```python
from build123d import *

# Parameters (mm, degrees)
SKETCH1_W           = 260
SKETCH1_H           = 170
BOSS_EXTRUDE1_DEPTH = 2
BOSS_EXTRUDE2_DEPTH = 3
CUT_EXTRUDE1_DEPTH  = 156.402702679
SKETCH4_R           = 2.5
CUT_EXTRUDE2_DEPTH  = 156.402702679
CUT_EXTRUDE3_REACH  = 157.403
SKETCH6_R           = 2.25


with BuildPart() as part:
    # Sketch1 → Boss-Extrude1 (new body)
    with BuildSketch(Plane.XY):
        Rectangle(SKETCH1_W, SKETCH1_H)
    extrude(amount=BOSS_EXTRUDE1_DEPTH)

    # Sketch2 → Boss-Extrude2 (add)
    with BuildSketch(Plane(origin=(0, 0, 0), x_dir=(-1, 0, 0), z_dir=(0, 0, -1))):
        with BuildLine():
            Line((-120.492, 81.492), (120.492, 81.492))
            Line((120.492, 81.492), (120.492, 79))
            ThreePointArc((120.492, 79), (121.519469412, 76.519469412), (124, 75.492))
            Line((124, 75.492), (126.492, 75.492))
            Line((126.492, 75.492), (126.492, -75.492))
            Line((126.492, -75.492), (124, -75.492))
            ThreePointArc((124, -75.492), (121.519469412, -76.519469412), (120.492, -79))
            Line((120.492, -79), (120.492, -81.492))
            Line((120.492, -81.492), (-120.492, -81.492))
            Line((-120.492, -81.492), (-120.492, -79))
            ThreePointArc((-120.492, -79), (-121.519469412, -76.519469412), (-124, -75.492))
            Line((-124, -75.492), (-126.492, -75.492))
            Line((-126.492, -75.492), (-126.492, 75.492))
            Line((-126.492, 75.492), (-124, 75.492))
            ThreePointArc((-124, 75.492), (-121.519469412, 76.519469412), (-120.492, 79))
            Line((-120.492, 79), (-120.492, 81.492))
        make_face()
    extrude(amount=BOSS_EXTRUDE2_DEPTH)

    # Sketch3 → Cut-Extrude1 (cut, through all)
    with BuildSketch(Plane.XY.offset(2)):
        with BuildLine():
            Line((-108.441183291, -1.769742849), (-108.441183291, -51.769742849))
            ThreePointArc((-108.441183291, -51.769742849), (-109.941183291, -53.269742849), (-111.441183291, -51.769742849))
            Line((-111.441183291, -51.769742849), (-111.441183291, -1.769742849))
            ThreePointArc((-111.441183291, -1.769742849), (-109.941183291, -0.269742849), (-108.441183291, -1.769742849))
        make_face()
        with BuildLine():
            Line((-103.441183291, -1.769742849), (-103.441183291, -51.769742849))
            ThreePointArc((-103.441183291, -51.769742849), (-104.941183291, -53.269742849), (-106.441183291, -51.769742849))
            Line((-106.441183291, -51.769742849), (-106.441183291, -1.769742849))
            ThreePointArc((-106.441183291, -1.769742849), (-104.941183291, -0.269742849), (-103.441183291, -1.769742849))
        make_face()
        with BuildLine():
            Line((-98.441183291, -1.769742849), (-98.441183291, -51.769742849))
            ThreePointArc((-98.441183291, -51.769742849), (-99.941183291, -53.269742849), (-101.441183291, -51.769742849))
            Line((-101.441183291, -51.769742849), (-101.441183291, -1.769742849))
            ThreePointArc((-101.441183291, -1.769742849), (-99.941183291, -0.269742849), (-98.441183291, -1.769742849))
        make_face()
        with BuildLine():
            Line((-93.441183291, -1.769742849), (-93.441183291, -51.769742849))
            ThreePointArc((-93.441183291, -51.769742849), (-94.941183291, -53.269742849), (-96.441183291, -51.769742849))
            Line((-96.441183291, -51.769742849), (-96.441183291, -1.769742849))
            ThreePointArc((-96.441183291, -1.769742849), (-94.941183291, -0.269742849), (-93.441183291, -1.769742849))
        make_face()
        with BuildLine():
            Line((-88.441183291, -1.769742849), (-88.441183291, -51.769742849))
            ThreePointArc((-88.441183291, -51.769742849), (-89.941183291, -53.269742849), (-91.441183291, -51.769742849))
            Line((-91.441183291, -51.769742849), (-91.441183291, -1.769742849))
            ThreePointArc((-91.441183291, -1.769742849), (-89.941183291, -0.269742849), (-88.441183291, -1.769742849))
        make_face()
        with BuildLine():
            Line((-83.441183291, -1.769742849), (-83.441183291, -51.769742849))
            ThreePointArc((-83.441183291, -51.769742849), (-84.941183291, -53.269742849), (-86.441183291, -51.769742849))
            Line((-86.441183291, -51.769742849), (-86.441183291, -1.769742849))
            ThreePointArc((-86.441183291, -1.769742849), (-84.941183291, -0.269742849), (-83.441183291, -1.769742849))
        make_face()
        with BuildLine():
            Line((-78.441183291, -1.769742849), (-78.441183291, -51.769742849))
            ThreePointArc((-78.441183291, -51.769742849), (-79.941183291, -53.269742849), (-81.441183291, -51.769742849))
            Line((-81.441183291, -51.769742849), (-81.441183291, -1.769742849))
            ThreePointArc((-81.441183291, -1.769742849), (-79.941183291, -0.269742849), (-78.441183291, -1.769742849))
        make_face()
    extrude(amount=-CUT_EXTRUDE1_DEPTH, mode=Mode.SUBTRACT)

    # Sketch4 → Cut-Extrude2 (cut, through all)
    with BuildSketch(Plane.XY.offset(2)):
        with Locations((110, -65)):
            Circle(SKETCH4_R)
    extrude(amount=-CUT_EXTRUDE2_DEPTH, mode=Mode.SUBTRACT)

    # Sketch6 → Cut-Extrude3 (cut, up to next)
    with BuildSketch(Plane.XY.offset(2), mode=Mode.PRIVATE) as cut_extrude3_sk1:
        with Locations((-125.5, -80.5)):
            Circle(SKETCH6_R)
    cut_extrude3_tool1 = extrude(cut_extrude3_sk1.sketch, amount=-CUT_EXTRUDE3_REACH, mode=Mode.PRIVATE) & part.part
    # Sketch6 → Cut-Extrude3 (cut, up to next)
    with BuildSketch(Plane.XY.offset(2), mode=Mode.PRIVATE) as cut_extrude3_sk2:
        with Locations((-125.5, 80.5)):
            Circle(SKETCH6_R)
    cut_extrude3_tool2 = extrude(cut_extrude3_sk2.sketch, amount=-CUT_EXTRUDE3_REACH, mode=Mode.PRIVATE) & part.part
    # Sketch6 → Cut-Extrude3 (cut, up to next)
    with BuildSketch(Plane.XY.offset(2), mode=Mode.PRIVATE) as cut_extrude3_sk3:
        with Locations((125.5, 80.5)):
            Circle(SKETCH6_R)
    cut_extrude3_tool3 = extrude(cut_extrude3_sk3.sketch, amount=-CUT_EXTRUDE3_REACH, mode=Mode.PRIVATE) & part.part
    # Sketch6 → Cut-Extrude3 (cut, up to next)
    with BuildSketch(Plane.XY.offset(2), mode=Mode.PRIVATE) as cut_extrude3_sk4:
        with Locations((125.5, -80.5)):
            Circle(SKETCH6_R)
    cut_extrude3_tool4 = extrude(cut_extrude3_sk4.sketch, amount=-CUT_EXTRUDE3_REACH, mode=Mode.PRIVATE) & part.part
    add(cut_extrude3_tool1.solids().sort_by_distance((-125.5, -80.5, 2))[0], mode=Mode.SUBTRACT)
    add(cut_extrude3_tool2.solids().sort_by_distance((-125.5, 80.5, 2))[0], mode=Mode.SUBTRACT)
    add(cut_extrude3_tool3.solids().sort_by_distance((125.5, 80.5, 2))[0], mode=Mode.SUBTRACT)
    add(cut_extrude3_tool4.solids().sort_by_distance((125.5, -80.5, 2))[0], mode=Mode.SUBTRACT)


solid = part.part
```
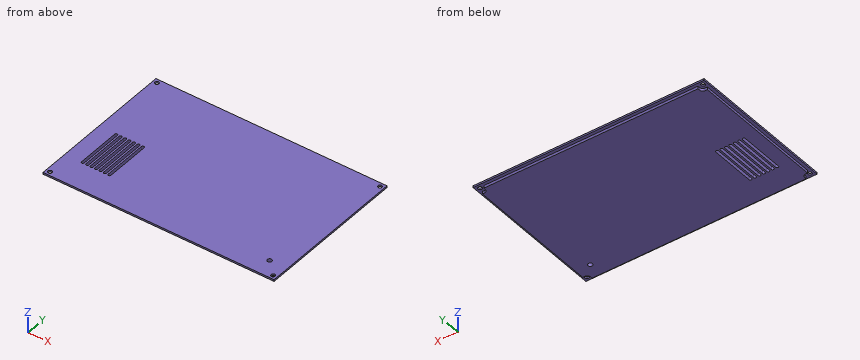
CAD build for the part. Positions are in the model's coordinates, mm. Coordinates: 2 decimals unless noted, no trailing zeros. Order: outer loops, then holes, each group sorted by start corner. A loop starts at its lowest first (then second) coordinate and runs counter-clockwise, first axis right, second up.
(1) Drill centre lines: L1, parallel to Y at x = -125.5, z = 1.05; L2, parallel to Y at x = 110, z = 1.4; L3, parallel to X at y = -59, z = -1.15. Where is each one in solid material? Low to high.
Solution:
L1: y = -85 to -82.75, -78.25 to 78.25, 82.75 to 85
L2: y = -85 to -67.5, -62.5 to 85
L3: x = -126.49 to 126.49
(2) Saw through at A-A, the plane x = 110. Write the cut outline in (y, z), and give its area (3 significant figures).
Solution:
outline: (-85, 0) - (-81.49, 0) - (-81.49, -3) - (-67.5, -3) - (-67.5, 2) - (-85, 2) - close; (-62.5, -3) - (81.49, -3) - (81.49, 0) - (85, 0) - (85, 2) - (-62.5, 2) - close
area: 804 mm2
(3) Pin check, flat tips, straight feed: pin 1 Ø1.5 at (y, z) = (33, -1) entering from +X; pin 2 Ø4.5 at (x, y) = (110, -65) entering from -Z; pin 3 Ø1.2 at (y, z) = (80, -1) entering from -X; pin 4 Ø1.2 at (x, z) = (125, -2) entering from -Y. Stop position of each tip, or through.
Solution:
pin 1: stops at x = 126.49
pin 2: passes through
pin 3: stops at x = -120.49
pin 4: stops at y = -75.49
(4) Saw through at C-C, the plane y = -20. Count the separate pieces of the cut face and the enclosed holes in it, and give its area (3 significant figures).
Solution:
separate pieces: 8
enclosed holes: 0
area: 1,170 mm2
(5) Saw through at B-B, the plane y = -65. Write the cut outline in (x, z), and give its area (3 significant figures).
Solution:
outline: (-130, 0) - (-126.49, 0) - (-126.49, -3) - (107.5, -3) - (107.5, 2) - (-130, 2) - close; (112.5, -3) - (126.49, -3) - (126.49, 0) - (130, 0) - (130, 2) - (112.5, 2) - close
area: 1,250 mm2
